Autodesk Inventor part; units mm, degrees
ref_plane "YZ Plane" through (0, 0, 0) normal (1, 0, 0) x (0, 1, 0)
ref_plane "XZ Plane" through (0, 0, 0) normal (0, 1, 0) x (-1, 0, 0)
ref_plane "XY Plane" through (0, 0, 0) normal (0, 0, 1) x (1, 0, 0)
sketch "Boceto1" plane through (0, 0, 0) normal (0, 0, 1) x (1, 0, 0)
  line L0 (-13.5, 62) -> (13.5, 62)
  line L1 (13.5, 62) -> (13.5, 0)
  line L2 (13.5, 0) -> (-13.5, 0)
  line L3 (-13.5, 0) -> (-13.5, 62)
  line L4 (0, 0) -> (0, 62) construction
  line L5 (0, 40.815) -> (8.5, 35.9075)
  line L6 (8.5, 35.9075) -> (8.5, 26.0925)
  line L7 (8.5, 26.0925) -> (0, 21.185)
  line L8 (0, 21.185) -> (-8.5, 26.0925)
  line L9 (-8.5, 26.0925) -> (-8.5, 35.9075)
  line L10 (-8.5, 35.9075) -> (0, 40.815)
  line L11 (-8.5, 35.9075) -> (-13.5, 35.9075) construction
  line L12 (8.5, 35.9075) -> (13.5, 35.9075) construction
  point P0 (0, 31)
  dimension "d20" = 17
  dimension "d21" = 5
  dimension "d22" = 27
  dimension "d23" = 62
extrude "Extrusión1" add sketch "Boceto1" along normal blind 6
sketch "Boceto2" plane through (0, 0, 0) normal (0, 0, -1) x (-1, 0, 0)
  line L0 (-8.5, 26.0925) -> (-8.5, 35.9075)
  line L1 (-8.5, 35.9075) -> (0, 40.815)
  line L2 (0, 40.815) -> (8.5, 35.9075)
  line L3 (8.5, 35.9075) -> (8.5, 26.0925)
  line L4 (8.5, 26.0925) -> (0, 21.185)
  line L5 (0, 21.185) -> (-8.5, 26.0925)
  line L6 (13.5, 62) -> (-13.5, 62)
  line L7 (-13.5, 62) -> (-13.5, 0)
  line L8 (-13.5, 0) -> (13.5, 0)
  line L9 (13.5, 0) -> (13.5, 62)
  point P0 (0, 0)
extrude "Extrusión2" add sketch "Boceto2" along normal blind 6 contours L0 L1 L2 L3 L4 L5 | L9 L8 L7 L6
sketch "Boceto3" plane through (0, 0, -6) normal (0, 0, -1) x (-1, 0, 0)
  line L0 (0, 0) -> (0, 62) construction
  line L1 (-13.5, 62) -> (13.5, 62)
  circle A0 centre (0, 31) radius 5.5
  dimension "d18" = 11
extrude "Extrusión3" cut sketch "Boceto3" against normal up to next
sketch "Boceto5" plane through (0, 0, 6) normal (0, 0, 1) x (1, 0, 0)
  line L0 (-13.5, 0) -> (-13.5, 62)
  line L1 (13.5, 62) -> (13.5, 0)
  line L2 (-13.5, 0) -> (13.5, 0)
  line L3 (13.5, 0) -> (13.5, 12)
  line L4 (13.5, 12) -> (-13.5, 12)
  line L5 (-13.5, 12) -> (-13.5, 0)
  line L6 (13.5, 62) -> (-13.5, 62)
  line L7 (-13.5, 62) -> (13.5, 62)
  line L8 (13.5, 62) -> (13.5, 50)
  line L9 (13.5, 50) -> (-13.5, 50)
  line L10 (-13.5, 50) -> (-13.5, 62)
  line L11 (-17.3027, 31) -> (12.0796, 31) construction
  line L12 (-8.5, 26.0925) -> (-8.5, 35.9075)
  point P0 (0, 0)
  point P1 (-8.5, 31)
  dimension "d24" = 12
extrude "Extrusión4" add sketch "Boceto5" along normal blind 115 contours L0 L4 L1 L2 | L0 L6 L1 L9
sketch "Boceto9" plane through (-13.5, 0, -6) normal (0, -1, 0) x (1, 0, 0)
  circle A0 centre (13.5, 110) radius 5
  line L0 (0, 127) -> (27, 127)
  line L1 (13.5, 110) -> (13.5, 115)
  line L2 (13.5, 115) -> (13.5, 127)
  line L3 (0, 127) -> (27, 127)
  point P0 (13.5, 6)
  dimension "d25" = 10
  dimension "d32" = 12
extrude "Extrusión8" cut sketch "Boceto9" against normal up to surface (12 mm away)
sketch "Boceto10" plane through (0, 0, -6) normal (0, 0, -1) x (-1, 0, 0)
  circle A0 centre (0, 31) radius 11
  circle A1 centre (0, 31) radius 5.5
  point P0 (0, 0)
  dimension "d29" = 22
extrude "Extrusión9" cut sketch "Boceto10" against normal blind 2.5
sketch "Boceto11" plane through (-13.5, 12, 6) normal (0, 1, 0) x (1, 0, 0)
  line L0 (21.5, -106) -> (5.5, -106) construction
  line L1 (5.5, -106) -> (5.5, -90) construction
  line L2 (5.5, -90) -> (21.5, -90) construction
  line L3 (21.5, -90) -> (21.5, -106) construction
  line L4 (5.5, -106) -> (21.5, -90) construction
  circle A0 centre (13.5, -98) radius 8 construction
  circle A1 centre (13.5, -98) radius 11.3137
  line L5 (27, 0) -> (27, -115)
  circle A2 centre (13.5, -98) radius 5
  point P0 (13.5, 6)
  dimension "d45" = 16
extrude "Extrusión10" cut sketch "Boceto11" against normal blind 3 contours A1 | A2
sketch "Boceto12" plane through (-13.5, 0, -6) normal (0, -1, 0) x (1, 0, 0)
  circle A0 centre (13.5, 110) radius 11.3137
  line L0 (0, 127) -> (0, 0)
  point P0 (13.5, 6)
extrude "Extrusión11" cut sketch "Boceto12" against normal blind 3
sketch "Boceto14" plane through (-13.5, 62, -6) normal (0, 1, 0) x (1, 0, 0)
  circle A0 centre (13.5, -110) radius 5
  circle A1 centre (13.5, -110) radius 5
  point P0 (13.5, -6)
  dimension "d38" = 10
extrude "Extrusión12" cut sketch "Boceto14" against normal up to next
sketch "Boceto15" plane through (-13.5, 50, 6) normal (0, -1, 0) x (1, 0, 0)
  circle A0 centre (13.5, 98) radius 5
  circle A1 centre (13.5, 98) radius 12
  point P0 (13.5, -6)
  dimension "d41" = 24
extrude "Extrusión13" cut sketch "Boceto15" against normal blind 8
fillet "Empalme4" radius 12 4 edges at (13.5, 56, 121) (-13.5, 56, 121) (13.5, 6, 121) (-13.5, 6, 121)
sketch "Boceto17" plane through (13.5, 12, 6) normal (1, 0, 0) x (0, 0, -1)
  line L0 (-103, 38) -> (-115, 38)
  line L1 (-103, 50) -> (12, 50)
  line L2 (-115, 38) -> (0, 38)
  line L3 (0, 38) -> (0, 50)
  line L4 (0, 50) -> (-115, 50)
  line L5 (-115, 50) -> (-115, 38)
  point P0 (6, -12)
extrude "Extrusión14" cut sketch "Boceto17" against normal up to next
fillet "Empalme7" radius 6 2 edges at (0, 62, -6) (0, 62, 6)
fillet "Empalme8" radius 27 1 edges at (0, 12, 6)
fillet "Empalme9" radius 27 1 edges at (0, 0, -6)
properties part number "U2"
Design review of the part built by this model. Coordinates are the model's own, in mm. A direction names the side the tool comes from. Give positions to 0.01 mm unless a question says otherwise; leave off trailing zeros. Write each loop counter-clockwise with the first axis right and the second up, starting at its lowest first coordinate (ties: lowest second). Pieces come first, ordered by that corner, then holes. Notation, with made-up numbers: M -16.5,30.25 L -11.5,30.25 A14 ccw -11.5,39.25 Z; hole C -6,63.25 d5. An arc over 180 degrees is marked long. Answer as a JSON object with one key per item and string values. Group by question number.
1) For line 1 along Z through (x, y) = (7.25, 56); line 2 along Z through (x, y) = (2, 37.5); line 3 along Y through (x, z) = (5.75, 42), list the stretches that pass through material, from the lowest coordinate up.
2) Mouldability with a two-part tool opening along Y and no side actions: class faces 1 (the face through (0, 0, 59)), 2 (the face through (0, 12, 67)), 3 (the face through (-1.08, 5.96, 99.12)), 4 (the face through (-8.5, 31, 4)) as released by +Y, released by -Y, zero draft, split by the parting line, or undercut.
3) We need section D-D (y = 49). Give the boundary of the cut face in (x, z).
4) We need section B-B (y = 31). Give the boundary of the cut face in (x, z), and give its area (3 significant figures).
5) Clearance check with flat-ended pins moving along their axes: pin 1 Ø1 at (x, y) = (0.5, 19.5) entering from -Z; pin 2 Ø7 at (x, z) = (-3.5, 109) entering from -Y; pin 3 Ø9 at (x, z) = (0, 104) entering from -Y; pin 4 Ø2 at (x, z) = (-4.5, 43.5) entering from +Y. State where each tip first meets the part, or that it passes through.
6) We need section C-C (y = 6.5). Give the boundary of the cut face in (x, z), and give its area (3 significant figures).
7) Tool access review of faces 5 (the face through (8.5, 31, 4)), 6 (the face through (-2.453, 10.521, 115.045)), 7 (the face through (1.432, 41.906, -4.768)), 8 (the face through (-2.453, 1.479, 92.955)): name each direction out of +Z, -Z, +X, -X, +Y, -Y from which nothing blocks a thin tool from reaching the whole face with its end or side.
8) We need section A-A (z = 104). Give the boundary of the cut face in (x, y).
Answer key:
{
 "1": {"line 1": "z = -6 to 6", "line 2": "z = -3.5 to 0", "line 3": "y = 0 to 12"},
 "2": {"face 1": "released by -Y", "face 2": "released by +Y", "face 3": "zero draft", "face 4": "undercut"},
 "3": {"outline": "M -13.5,-6 L 13.5,-6 L 13.5,6 L -13.5,6 Z"},
 "4": {"outline": "M -13.5,-6 L -11,-6 L -11,-3.5 L -5.5,-3.5 L -5.5,0 L -8.5,0 L -8.5,7.21 L -13.5,7.21 Z; M 5.5,-3.5 L 11,-3.5 L 11,-6 L 13.5,-6 L 13.5,7.21 L 8.5,7.21 L 8.5,0 L 5.5,0 Z", "area": "141 mm²"},
 "5": {"pin 1": "stops at z = -5.08", "pin 2": "stops at y = 3", "pin 3": "passes through", "pin 4": "stops at y = 12"},
 "6": {"outline": "M -13.5,3.43 L 13.5,3.43 L 13.5,109 A12 ccw 1.5,121 L -1.5,121 A12 ccw -13.5,109 Z; hole C 0,104 d10", "area": "3,030 mm²"},
 "7": {"face 5": "+Z", "face 6": "+Y", "face 7": "-Z", "face 8": "-Y"},
 "8": {"outline": "M -13.5,0 L -11.31,0 L -11.31,3 L -5,3 L -5,9 L -11.31,9 L -11.31,12 L -13.5,12 Z; M 5,3 L 11.31,3 L 11.31,0 L 13.5,0 L 13.5,12 L 11.31,12 L 11.31,9 L 5,9 Z"}
}
